Source: CAD feature listing. Evaluate the final solid. Frame: model axes, mm. A direction names the side the tool comes from. Round coordinates to 2 decimals unless told otherwise and drop trailing zeros. Order: outer loops, then holes, each group sorted by start corner. A loop starts at its lowest first (then second) coordinate and runs counter-clockwise, first axis right, second up. Notation, with made-up numbers: M -31,49.5 L 22,49.5 A26 cw 22,79.5 Z; hole C 84.5,-33 d10. An arc over 180 degrees is marked long. Use CSV: the item, a comma, the result in double quotes. Start each with the question number.
```python
from build123d import *

# Parameters (mm, degrees)
SKETCH_1_W          = 57
SKETCH_1_H          = 57
EXTRUDE_1_DEPTH     = 4.5
FILLET_1_R          = 3
SKETCH_2_R          = 19
EXTRUDE_2_DEPTH     = 2
EXTRUDE_3_DEPTH     = 26
SKETCH_4_R          = 2.75
CUT_EXTRUDE_1_DEPTH = 15
SKETCH_5_R          = 28.5
EXTRUDE_4_DEPTH     = 10
SKETCH_6_R          = 27.5
EXTRUDE_5_DEPTH     = 20
SKETCH_7_R          = 28.5
EXTRUDE_6_DEPTH     = 20


with BuildPart() as part:
    # 草图1 → 凸台-拉伸1 (new body)
    with BuildSketch(Plane.XY):
        Rectangle(SKETCH_1_W, SKETCH_1_H)
    extrude(amount=EXTRUDE_1_DEPTH)

    # 圆角1
    fillet_1_edges = [part.edges().sort_by_distance(p)[0] for p in [
        (28.5, -28.5, 2.25),
        (-28.5, -28.5, 2.25),
        (-28.5, 28.5, 2.25),
        (28.5, 28.5, 2.25),
    ]]
    fillet(fillet_1_edges, radius=FILLET_1_R)

    # 草图2 → 凸台-拉伸2 (add)
    with BuildSketch(Plane.XY.offset(4.5)):
        Circle(SKETCH_2_R)
    extrude(amount=EXTRUDE_2_DEPTH)

    # 草图3 → 凸台-拉伸3 (add)
    with BuildSketch(Plane.XY.offset(6.5)):
        with BuildLine():
            Line((-1.25, 3.799671038), (-1.25, 5.299671038))
            Line((-1.25, 5.299671038), (1.25, 5.299671038))
            Line((1.25, 5.299671038), (1.25, 3.799671038))
            ThreePointArc((1.25, 3.799671038), (0, -4), (-1.25, 3.799671038))
        make_face()
    extrude(amount=EXTRUDE_3_DEPTH)

    # 草图4 → 切除-拉伸1 (cut)
    with BuildSketch(Plane.XY.offset(4.5)):
        with Locations((-23.5, 23.5)):
            Circle(SKETCH_4_R)
        with Locations((23.5, 23.5)):
            Circle(SKETCH_4_R)
        with Locations((-23.5, -23.5)):
            Circle(SKETCH_4_R)
        with Locations((23.5, -23.5)):
            Circle(SKETCH_4_R)
    extrude(amount=-CUT_EXTRUDE_1_DEPTH, mode=Mode.SUBTRACT)

    # 草图5 → 凸台-拉伸4 (add)
    with BuildSketch(Plane(origin=(0, 0, 0), x_dir=(-1, 0, 0), z_dir=(0, 0, -1))):
        Circle(SKETCH_5_R)
    extrude(amount=EXTRUDE_4_DEPTH)

    # 草图6 → 凸台-拉伸5 (add)
    with BuildSketch(Plane(origin=(0, 0, -10), x_dir=(-1, 0, 0), z_dir=(0, 0, -1))):
        Circle(SKETCH_6_R)
    extrude(amount=EXTRUDE_5_DEPTH)

    # 草图7 → 凸台-拉伸6 (add)
    with BuildSketch(Plane(origin=(0, 0, -30), x_dir=(-1, 0, 0), z_dir=(0, 0, -1))):
        Circle(SKETCH_7_R)
    extrude(amount=EXTRUDE_6_DEPTH)


solid = part.part
```
(1) Section D-D on x = -16. Return loops of the section in (y, z).
(2) Section B-B on x = -24. Return loops of the section in (y, z).
(3) Reachability of faces 5 (the face through (-19.4, 0.4, 4.5)), 6 (the face through (-26.327, -10.916, -4.93)), 7 (the face through (21, 22, 0)), 8 (the face through (-22, -21, 0)) from +Z, -Z, +X, -X, +Y, -Y: full face, straight path, thin tool, end or side. Return the list, or none.
(4) Line query: line 1 along Y through (x, z) = (23.5, 1.65); line 2 along X through (y, z) = (23, 1); line 3 along Z through (x, y) = (3, -14). Output: solid intervals per line, ascending.
(5) Section C-C on y = -14. Return loops of the section in (x, z), plus the area to 3 significant figures.
(6) Section A-A on y = -23.5. Return loops of the section in (x, z), plus the area to 3 significant figures.
(7) Draft query along Z for faces 1 (the face through (-22.8, 20.6, 0)), 2 (the face through (20.753, 23.621, 2.282)), 3 (the face through (14.9, 23.4, -30)), 4 (the face through (5.961, -26.846, -19.86)). Return one class per face: pulls with the +Z half, pulls with the -Z half, needs draft (parallel to the pull), parting line crosses it, or undercut.
(8) Contact query for flat-ended pins moving along their axis: P1, Ø2, axis at x = 0.5, z = 21, coming from the +Y side; P2, Ø1.5, axis at y = -10, z = -4.5, coming from the -X side; P3, Ø1, axis at x = 5, z = -13, coming from the -Y side. Output: stop coordinate, or through.
Results below:
1,outline,"M -28.5,0 L -23.58,0 L -23.58,-10 L -22.37,-10 L -22.37,-30 L -23.58,-30 L -23.58,-50 L 23.58,-50 L 23.58,-30 L 22.37,-30 L 22.37,-10 L 23.58,-10 L 23.58,0 L 28.5,0 L 28.5,4.5 L 10.25,4.5 L 10.25,6.5 L -10.25,6.5 L -10.25,4.5 L -28.5,4.5 Z"
2,outline,"M -28.5,0 L -26.2,0 L -26.2,4.5 L -28.5,4.5 Z; M -20.8,0 L -15.37,0 L -15.37,-10 L -13.43,-10 L -13.43,-30 L -15.37,-30 L -15.37,-50 L 15.37,-50 L 15.37,-30 L 13.43,-30 L 13.43,-10 L 15.37,-10 L 15.37,0 L 20.8,0 L 20.8,4.5 L -20.8,4.5 Z; M 26.2,0 L 28.5,0 L 28.5,4.5 L 26.2,4.5 Z"
3,face 5,"+Z"
3,face 6,"-Z"
3,face 7,"-Z, +X, +Y"
3,face 8,"-Z, -X, -Y"
4,line 1,"y = -28.5 to -26.25, -20.75 to 20.75, 26.25 to 28.5"
4,line 2,"x = -28.5 to -26.2, -20.8 to 20.8, 26.2 to 28.5"
4,line 3,"z = -50 to 6.5"
5,outline,"M -28.5,0 L -24.82,0 L -24.82,-10 L -23.67,-10 L -23.67,-30 L -24.82,-30 L -24.82,-50 L 24.82,-50 L 24.82,-30 L 23.67,-30 L 23.67,-10 L 24.82,-10 L 24.82,0 L 28.5,0 L 28.5,4.5 L 12.85,4.5 L 12.85,6.5 L -12.85,6.5 L -12.85,4.5 L -28.5,4.5 Z"
5,area,"2,740 mm2"
6,outline,"M -28.5,0 L -26.25,0 L -26.25,4.5 L -28.5,4.5 Z; M -20.75,0 L -16.12,0 L -16.12,-10 L -14.28,-10 L -14.28,-30 L -16.12,-30 L -16.12,-50 L 16.12,-50 L 16.12,-30 L 14.28,-30 L 14.28,-10 L 16.12,-10 L 16.12,0 L 20.75,0 L 20.75,4.5 L -20.75,4.5 Z; M 26.25,0 L 28.5,0 L 28.5,4.5 L 26.25,4.5 Z"
6,area,"1,750 mm2"
7,face 1,"pulls with the -Z half"
7,face 2,"needs draft"
7,face 3,"undercut"
7,face 4,"undercut"
8,P1,"stops at y = 5.3"
8,P2,"stops at x = -26.96"
8,P3,"stops at y = -27.13"
